Verification items for the finished model (mm, model axes). Coordinates: 2 decimals unless noted, no trailing zeros. Order: outer loops, then holes, each group sorted by start corner. A loop starts at its lowest first (then second) coordinate and runs counter-clockwise, first axis right, second up. Notation, with made-up numbers: M -15.5,0 L 36.5,0 A16 cw 36.5,10 Z; hole C 24.5,76 d7. An arc over 180 degrees is marked long. Return JSON: item names as keys, results as strings.
```python
from build123d import *

# Parameters (mm, degrees)
F0_W      = 454.152
F0_H      = 1930.4
F1_DEPTH  = 19.05
F1_FACE_W = 454.152
F1_FACE_H = 19.05
F2_DEPTH  = 53.975
F4_DEPTH  = 25.4


with BuildPart() as f1:
    # F0 (on Front) → F1 (new body)
    with BuildSketch(Plane.XZ):
        Rectangle(F0_W, F0_H)
    extrude(amount=F1_DEPTH)

    # F1_face (on face) → F2 (cut)
    with BuildSketch(Plane(origin=(0, -9.525, -965.2), x_dir=(1, 0, 0), z_dir=(0, 0, -1))):
        Rectangle(F1_FACE_W, F1_FACE_H)
    extrude(amount=-F2_DEPTH, mode=Mode.SUBTRACT)

    # F3 (on face) → F4 (cut)
    with BuildSketch(Plane.XZ.offset(19.05)):
        Polygon((-111.125, -717.55), (0, -717.55), (111.125, -717.55), (111.125, -647.7), (-111.125, -647.7), align=None)
    extrude(amount=-F4_DEPTH, mode=Mode.SUBTRACT)


solid = f1.part
```
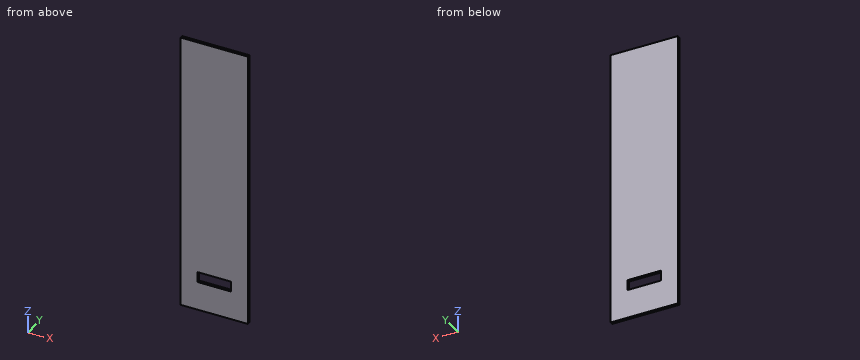
Q1. Cross-section at B-B, the plane x = -45.5. Record the boundary of the cut face in (y, z) (3 decimals), and give its area (3 significant figures).
Values:
{"outline": "M -19.05,-911.225 L 0,-911.225 L 0,-717.55 L -19.05,-717.55 Z; M -19.05,-647.7 L 0,-647.7 L 0,965.2 L -19.05,965.2 Z", "area": "34,400 mm^2"}
Q2. Cross-section at A-A, the plane y = -10. Record the boundary of the cut face in (x, z) (3 decimals).
Values:
{"outline": "M -227.076,-911.225 L 227.076,-911.225 L 227.076,965.2 L -227.076,965.2 Z; hole M -111.125,-717.55 L 111.125,-717.55 L 111.125,-647.7 L -111.125,-647.7 Z"}
Q3. Material ranges on line 1 along Z through (x, y) = (-67, -1.5) (3 decimals), recorded low to high.
Values:
{"line 1": "-911.225 to -717.55, -647.7 to 965.2"}
Q4. Go/stop test with a flat-tipped pin: pin 1 (4 mm diameter, centred on x = -127, z = 215, fed in from +Y). Record where the tip stops, or that it passes through.
Values:
{"pin 1": "y = 0"}
